from build123d import *

# Parameters (mm, degrees)
SKETCH_1_R      = 22.071639064
SKETCH_1_R_2    = 2.5
SKETCH_1_W      = 19
SKETCH_1_H      = 6
EXTRUDE_1_DEPTH = 5


with BuildPart() as part:
    # 스케치1 → 보스-돌출1 (new body)
    with BuildSketch(Plane.XY):
        Circle(SKETCH_1_R)
        with Locations((0, 12.45)):
            Circle(SKETCH_1_R_2, mode=Mode.SUBTRACT)
        with Locations((10.782016277, -6.225)):
            Circle(SKETCH_1_R_2, mode=Mode.SUBTRACT)
        with Locations((-10.782016277, -6.225)):
            Circle(SKETCH_1_R_2, mode=Mode.SUBTRACT)
        Rectangle(SKETCH_1_W, SKETCH_1_H, mode=Mode.SUBTRACT)
    extrude(amount=EXTRUDE_1_DEPTH)


solid = part.part
The model under review builds one solid part; all positions refer to its coordinate system, in mm. A direction names the side the tool comes from. Give positions to 0.01 mm unless a question says otherwise; leave off trailing zeros. Write each loop counter-clockwise with the first axis right and the second up, starting at its lowest first coordinate (ties: lowest second). Pieces come first, ordered by that corner, then holes. Notation, with made-up numbers: M 70,16.25 L 110,16.25 A20 cw 110,54.25 Z; hole C -39,27 d3. An arc over 180 degrees is marked long. One line per question, with ' | ' between items. Start each with the question number.
Item 1: Wall thickness on line 1 (Y direction, x = 0, z = 4); line 2 (X direction, y = -6, z = 1.75); line 3 (X direction, y = -4, z = 1.55): over which ranges is each line inside the solid? List them lowest first. Write a range as from..to.
Item 2: We need section A-A on x = 0. Write out the cut boundary in (y, z).
Item 3: Draft analysis for pull direction X (two halves, no side actions). For faces 3 (the flat face through (0, -5, 0)), 4 (the cylindrical face through (-4.785, -21.547, 2.465)), 5 (the flat face through (9.5, 0, 2)), 6 (the cylindrical face through (13.167, -5.474, 2.465)), state which applies: released by +X, released by -X, zero draft, split by the parting line, or undercut.
Item 4: We need section D-D on z = 1.5. Write out the cut boundary in (x, y) (3 decimals).
Item 5: For faces 1 (the flat face through (0, -5, 5)), 2 (the flat face through (-9.5, 0, 2)), list the 3-axis set-ups (+Z, -Z, +X, -X, +Y, -Y) from which the entire face can be reached by the end or side of a thin tool; tool diameter is ignored.
Item 6: We need section B-B on y = 0. Write out the cut boundary in (x, z), plus the area to 3 significant figures.
Item 7: We need section C-C on x = -12. Write out the cut boundary in (y, z), plus the area to 3 significant figures.
Item 8: For pin 1 (6 mm diameter, centred on x = 10.78, y = -6.22, fed in from -Z); pin 2 (4 mm diameter, centred on x = -10.78, y = -6.22, fed in from +Z); pin 3 (2 mm diameter, centred on y = -5, z = 2.5, fed in from +X); pin 4 (1 mm diameter, centred on x = -13, z = 1.5, fed in from -Y), all flat-tipped, find the tip position at first contact; note any pin that passes through.
Results found:
1) line 1: y = -22.07..-3, 3..9.95, 14.95..22.07 | line 2: x = -21.24..-13.27, -8.29..8.29, 13.27..21.24 | line 3: x = -21.71..-11.92, -9.64..9.64, 11.92..21.71
2) outline: M -22.07,0 L -3,0 L -3,5 L -22.07,5 Z; M 3,0 L 9.95,0 L 9.95,5 L 3,5 Z; M 14.95,0 L 22.07,0 L 22.07,5 L 14.95,5 Z
3) face 3: zero draft | face 4: split by the parting line | face 5: undercut | face 6: undercut
4) outline: C 0,0 d44.143; hole C -10.782,-6.225 d5; hole M -9.5,-3 L 9.5,-3 L 9.5,3 L -9.5,3 Z; hole C 0,12.45 d5; hole C 10.782,-6.225 d5
5) face 1: +Z, +X, -X, +Y, -Y | face 2: +Z, -Z
6) outline: M -22.07,0 L -9.5,0 L -9.5,5 L -22.07,5 Z; M 9.5,0 L 22.07,0 L 22.07,5 L 9.5,5 Z | area: 126 mm2
7) outline: M -18.52,0 L -8.41,0 L -8.41,5 L -18.52,5 Z; M -4.04,0 L 18.52,0 L 18.52,5 L -4.04,5 Z | area: 163 mm2
8) pin 1: stops at z = 0 | pin 2: passes through | pin 3: stops at x = 21.71 | pin 4: stops at y = -18.19
